Design review of the part built by this model. Coordinates are the model's own, in mm. Face numbers are marked on the shaded views. A direction names the side the tool comes from. Give positions to 0.01 mm unless a question says otherwise; leave off trailing zeros. Order: outer loops, then holes, each group sorted by start corner. A loop starts at its lowest first (then second) coordinate and runs counter-clockwise, first axis right, second up. Notation, with made-up numbers: (6.25, 25.5) -> (55.25, 25.5) arc R16 cw to (55.25, 56.5) -> close; hole circle Ø8 at (59, -13). An arc over 180 degrees is marked (long way). One line per item, written item: value.
from build123d import *

# Parameters (mm, degrees)
SKETCH_1_R              = 1.6
EXTRUDE_1_DEPTH         = 4
SHEET_METAL_1_OUTLINE_R = 1.6
SHEET_METAL_1_DEPTH     = 1


# Read off the part's stored shape, not the designer's step: 轉換-實體1
with BuildPart() as part:
    # Sketch 1 → 填料-伸長1 (new body)
    # profile 1 of 3: a face of its own
    with BuildSketch(Plane.XY):
        with BuildLine():
            ThreePointArc((-4, 0), (-2.828427125, 2.828427125), (0, 4))
            Line((0, 4), (4, 4))
            Line((4, 4), (4, 16.17))
            ThreePointArc((4, 16.17), (0, 20.17), (-4, 16.17))
            Line((-4, 16.17), (-4, 0))
        make_face()
        with Locations((0, 16.17)):
            Circle(SKETCH_1_R, mode=Mode.SUBTRACT)
    # profile 2 of 3: a face of its own
    with BuildSketch(Plane.XY):
        with BuildLine():
            Line((4, 4), (0, 4))
            ThreePointArc((0, 4), (-2.828427125, 2.828427125), (-4, 0))
            ThreePointArc((-4, 0), (-2.828427125, -2.828427125), (0, -4))
            ThreePointArc((0, -4), (2.828427125, -2.828427125), (4, 0))
            Line((4, 0), (4, 4))
        make_face()
    # profile 3 of 3: a face of its own
    with BuildSketch(Plane.XY):
        with BuildLine():
            Line((19.08, 4), (4, 4))
            Line((4, 4), (4, 0))
            ThreePointArc((4, 0), (2.828427125, -2.828427125), (0, -4))
            Line((0, -4), (19.08, -4))
            ThreePointArc((19.08, -4), (23.08, 0), (19.08, 4))
        make_face()
        with Locations((9.08, 0)):
            Circle(SKETCH_1_R, mode=Mode.SUBTRACT)
        with Locations((19.08, 0)):
            Circle(SKETCH_1_R, mode=Mode.SUBTRACT)
    extrude(amount=EXTRUDE_1_DEPTH)

    # Sheet Metal 1 outline → Sheet Metal 1 (cut)
    with BuildSketch(Plane.XY):
        with BuildLine():
            ThreePointArc((4, 16.17), (0, 20.17), (-4, 16.17))
            Line((-4, 16.17), (-4, 0))
            ThreePointArc((-4, 0), (-2.828427125, -2.828427125), (0, -4))
            Line((0, -4), (19.08, -4))
            ThreePointArc((19.08, -4), (23.08, 0), (19.08, 4))
            Line((19.08, 4), (4, 4))
            Line((4, 4), (4, 16.17))
        make_face()
        with Locations((9.08, 0)):
            Circle(SHEET_METAL_1_OUTLINE_R, mode=Mode.SUBTRACT)
        with Locations((19.08, 0)):
            Circle(SHEET_METAL_1_OUTLINE_R, mode=Mode.SUBTRACT)
        with Locations((0, 16.17)):
            Circle(SHEET_METAL_1_OUTLINE_R, mode=Mode.SUBTRACT)
    extrude(amount=SHEET_METAL_1_DEPTH, mode=Mode.SUBTRACT)


solid = part.part
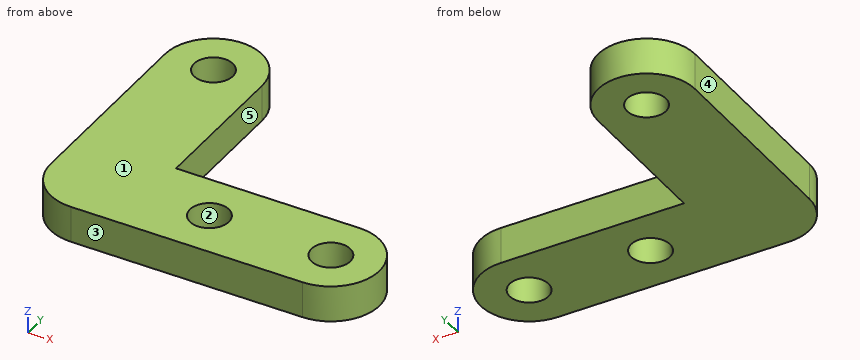
Item 1: Machinability: for the marked faces 4 and 5, which of the approach directions +Z, -Z, +X, -X, +Y, -Y give a long, thin tool a straight path to every point of the face, cutting with its end or side? Answer none if there is none.
Returned:
face 4: +Z, -Z, -X, +Y, -Y
face 5: +Z, -Z, +X, +Y
Item 2: To check wall thickness, follow line 1 along Y through (x, z) = (9.08, 2.9); line 2 along Y through (x, z) = (0, 1.8); line 3 along X through (y, z) = (-0.5, 2.15). State the ranges of each line that lie inside material, in increasing order. Write a range as from..to.
Returned:
line 1: -4..-1.6, 1.6..4
line 2: -4..14.57, 17.77..20.17
line 3: -3.97..7.56, 10.6..17.56, 20.6..23.05
Item 3: Add section D-D on y = 14.25. Give the boundary of the cut face in (x, z), plus the area to 3 significant figures.
Returned:
outline: (-4, 1) -> (4, 1) -> (4, 4) -> (-4, 4) -> close
area: 24.0 mm²
Item 4: Add section B-B on z = 2.75. Give the boundary of the cut face in (x, y).
Returned:
outline: (-4, 0) arc R4 ccw to (0, -4) -> (19.08, -4) arc R4 ccw to (19.08, 4) -> (4, 4) -> (4, 16.17) arc R4 ccw to (-4, 16.17) -> close; hole circle Ø3.2 at (0, 16.17); hole circle Ø3.2 at (9.08, 0); hole circle Ø3.2 at (19.08, 0)
Item 5: Add section A-A on x = 9.08. Give the boundary of the cut face in (y, z).
Returned:
outline: (-4, 1) -> (-1.6, 1) -> (-1.6, 4) -> (-4, 4) -> close; (1.6, 1) -> (4, 1) -> (4, 4) -> (1.6, 4) -> close
Item 6: Clearance check with flat-ended pins moving along their axes: P1, Ø0.9, axis at x = 15, z = 2, coming from the +Y side; P2, Ø1.5, axis at y = 14.5, z = 2.5, coming from the +X side; P3, Ø1.5, axis at x = 1, z = 1.5, coming from the +Y side. State where each tip first meets the part, or that it passes through.
Returned:
P1: y = 4
P2: x = 4
P3: y = 20.16
Item 7: Draft analysis for pull direction Y (two halves, no side actions). For the marked faces 1, 2 and 3, state which applies: pulls with the +Y half, pulls with the -Y half, needs draft (parallel to the pull), parting line crosses it, or undercut.
Returned:
face 1: needs draft
face 2: undercut
face 3: pulls with the -Y half
Item 8: Add section C-C on x = 18. Give the boundary of the cut face in (y, z), plus the area to 3 significant figures.
Returned:
outline: (-4, 1) -> (-1.18, 1) -> (-1.18, 4) -> (-4, 4) -> close; (1.18, 1) -> (4, 1) -> (4, 4) -> (1.18, 4) -> close
area: 16.9 mm²
